The figure shows three views and two pictorial views of one solid part (mm, origin at its lowest corner). Answer the questions. Coordinates: 2 decimals unless noted, no trailing zeros. Loops run counter-clockwise (first coordinate to the right, second up) from the corner with the lowest first, then second, coordinate; pieces in that order, holes last.
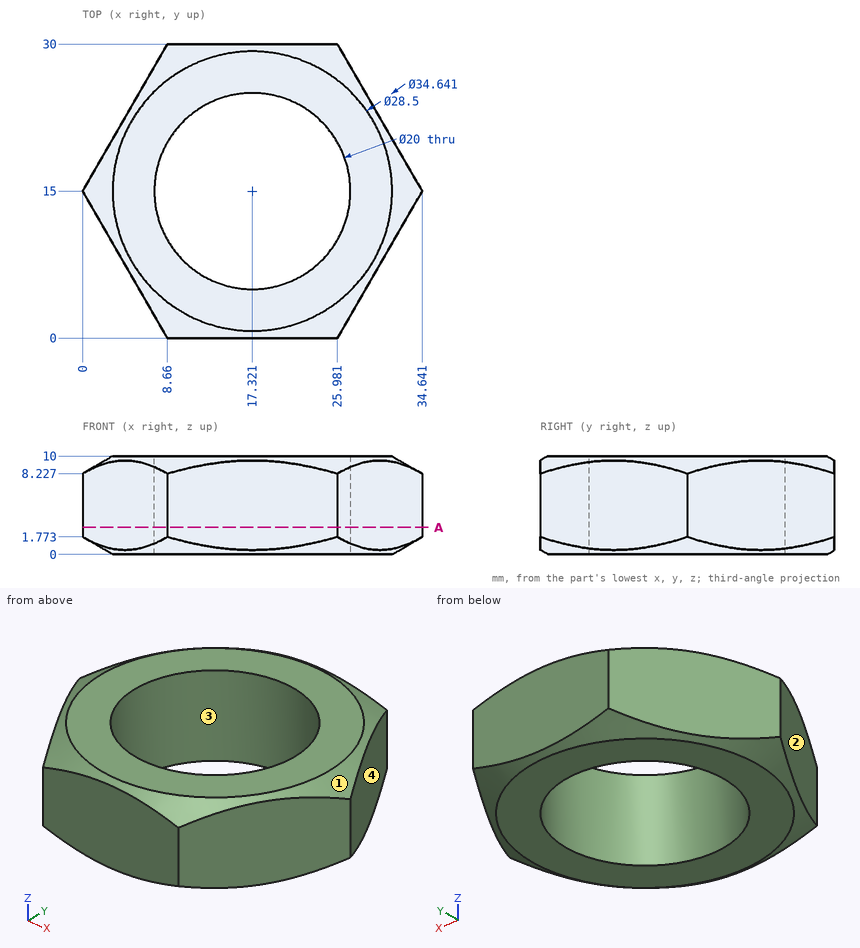
Q1. Straight lines are drawn through the part: probe 1 along Y at (x, z) = (9.5, 7.25) (1 decimal); probe 2 along X at (y, z) = (17, 3.75) (1 decimal); probe 3 along Y at (x, z) = (17, 2.5) (1 decimal). For each, find the intervals that lie inside material, in ascending order.
Findings below:
probe 1: y = 0 to 8.8, 21.2 to 30
probe 2: x = 1.2 to 7.5, 27.1 to 33.5
probe 3: y = 0 to 5, 25 to 30
Q2. Determine the mould class of the marked faces 1, 2, 3 and 4 for opening direction Y: +Y half, -Y half, draft (parallel to the pull), parting line (faces both ways), or undercut.
Findings below:
face 1: parting line
face 2: -Y half
face 3: undercut
face 4: +Y half
Q3. Flat-ended cylindrical pins translate along their axes: pin 1 Ø1.5 at (y, z) = (13.5, 5) entering from -X; pin 2 Ø2 at (x, y) = (24.5, 10) entering from -Z; pin 3 Ø3 at (x, z) = (4, 6.5) entering from -Y (1 decimal); pin 4 Ø1.5 at (y, z) = (16.5, 1.5) entering from +X. Find the tip coordinate at first contact, or state that the pin passes through.
Findings below:
pin 1: stops at x = 0.43
pin 2: passes through
pin 3: stops at y = 5.5
pin 4: stops at x = 34.21
Q4. A cutting plane is placed at A-A (z = 2.75). Give the vertices of the cut face in (x, y), then the cut area to 3 significant figures.
Findings below:
outline: (0, 15) - (8.66, 0) - (25.98, 0) - (34.64, 15) - (25.98, 30) - (8.66, 30) - close; hole circle Ø20 at (17.32, 15)
area: 465 mm2
